The listing builds one solid part. Answer for the finished solid, in the listing's coordinates (mm). Face numbers are marked on the shaded views. A direction names the side the tool comes from. Coordinates: 2 decimals unless noted, no trailing zeros. Loops run counter-clockwise (first coordinate to the right, second up) from the corner with the lowest first, then second, coordinate; pieces in that order, holes last. Notation, with made-up numbers: (36, 69.5) - (79, 69.5) arc R7 ccw to (79, 78.5) - close; hole circle Ø7 at (40, 84.5). An arc over 180 degrees is marked (long way). Put each result on its own line as item: value.
```python
from build123d import *

# Parameters (mm, degrees)
F2_T     = -2.5
F3_W     = 54.863745
F3_H     = 16.608417
F4_DEPTH = 104.5
F5_W     = 77.0705
F5_H     = 24.25948
F6_DEPTH = 90.4
F8_W     = 123.194821
F8_H     = 89.151054
F9_DEPTH = 91.698781


with BuildPart() as f1:
    # F0 (on Front) → F1 (revolve)
    with BuildSketch(Plane.XZ):
        Polygon((0, 44.082265), (0, 0), (60.916152, 32.297436), (60.916152, 44.082265), align=None)
    revolve(axis=Axis((0, 0, 22.041133), (0, 0, 1)))

    # F2
    f2_openings = [f1.faces().sort_by_distance(p)[0] for p in [
        (0, 0, 44.082265),
    ]]
    offset(amount=F2_T, openings=f2_openings)

    # F3 (on Front) → F4 (cut, symmetric)
    with BuildSketch(Plane.XZ):
        with Locations((-2.892476, 45.159954)):
            Rectangle(F3_W, F3_H)
    extrude(amount=F4_DEPTH, both=True, mode=Mode.SUBTRACT)

    # F5 (on Right) → F6 (cut, symmetric)
    with BuildSketch(Plane.YZ):
        with Locations((-2.79917, -1.772808)):
            Rectangle(F5_W, F5_H)
    extrude(amount=F6_DEPTH, both=True, mode=Mode.SUBTRACT)

    # F8 (on face) → F9 (join)
    with BuildSketch(Plane.XY):
        with Locations((-12.236293, 9.672433)):
            Rectangle(F8_W, F8_H)
    extrude(amount=F9_DEPTH)


solid = f1.part
```
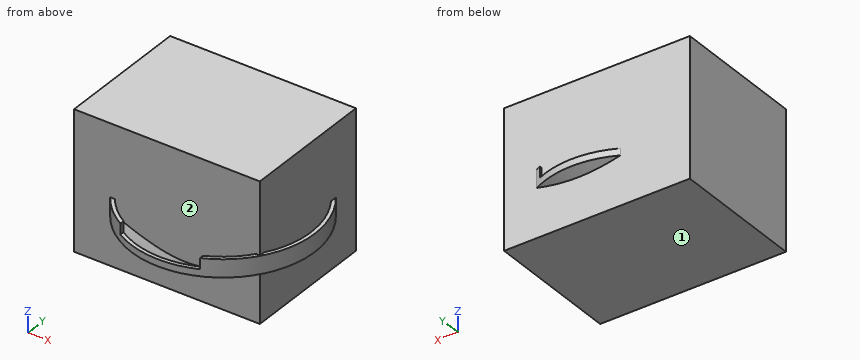
1) The part is cut by section C-C (y = 0). Give the vertices of the cut face in (x, z).
Found:
outline: (-73.83, 0) - (49.36, 0) - (49.36, 26.17) - (60.92, 32.3) - (60.92, 44.08) - (58.42, 44.08) - (58.42, 33.8) - (49.36, 29) - (49.36, 91.7) - (-73.83, 91.7) - close
2) The part is cut by section D-D (x = -54). Give the vertices of the cut face in (y, z), and give its area (3 significant figures).
Found:
outline: (-34.9, 0) - (54.25, 0) - (54.25, 91.7) - (-34.9, 91.7) - close
area: 8,180 mm^2
3) Straight lines are drawn through the part: L1, parallel to Y at x = 28, z = 45; L2, parallel to Y at x = 36, z = 40.5; L3, parallel to X at y = 49.5, z = 20. For each, find the intervals that lie inside material, in ascending order. Write a range as [from, to].
Found:
L1: y = [-34.9, 54.25]
L2: y = [-49.14, -46], [-34.9, 54.25]
L3: x = [-73.83, 49.36]
4) The part is cut by section B-B (z = 71). Give the vertices of the cut face in (x, y).
Found:
outline: (-73.83, -34.9) - (49.36, -34.9) - (49.36, 54.25) - (-73.83, 54.25) - close
5) For the marked faces 1 and 2, determine the directions among +Z, -Z, +X, -X, +Y, -Y from which every point of the face is accessible in a straight line to the end or side of a thin tool.
Found:
face 1: -Z, +X, -X, +Y, -Y
face 2: none
6) The part is cut by section A-A (x = 0). Give the vertices of the cut face in (y, z).
Found:
outline: (-60.92, 32.3) - (-34.9, 18.51) - (-34.9, 0) - (54.25, 0) - (54.25, 28.76) - (60.92, 32.3) - (60.92, 36.86) - (58.42, 36.86) - (58.42, 33.8) - (54.25, 31.59) - (54.25, 91.7) - (-34.9, 91.7) - (-34.9, 21.34) - (-58.42, 33.8) - (-58.42, 36.86) - (-60.92, 36.86) - close
7) Each of these flat-tipped pins is pushed along its axis until it touches: pin 1 (9 mm diameter, centred on x = -13.5, y = -55, fed in from +Z); pin 2 (10 mm diameter, centred on y = -38.5, z = 47.5, fed in from +X); pin 3 (3 mm diameter, centred on y = -55, z = 39.5, fed in from -X); pin 4 (19.5 mm diameter, centred on x = -43.5, y = -41.5, fed in from +Z). Where does it stop, or does it pass through?
Found:
pin 1: stops at z = 36.86
pin 2: stops at x = 49.96
pin 3: stops at x = 24.54
pin 4: stops at z = 91.7
